The listing builds one solid part. Answer for the finished solid, in the listing's coordinates (mm). A direction names the side the tool comes from. Coordinates: 2 decimals unless noted, no trailing zeros. Order: outer loops, then holes, each group sorted by start corner. A loop starts at its lowest first (then second) coordinate and runs counter-clockwise, first axis right, second up. Notation, with made-up numbers: (-23, -25) -> (18, -25) arc R6 ccw to (18, -19) -> close; hole circle Ø3 at (82.5, 51). An arc over 180 degrees is marked (long way). One line per question, with ' | ' between items.
from build123d import *

# Parameters (mm, degrees)
SKICA1_W                      = 160
SKICA1_H                      = 46
P_IDAT_VYSUNUT_M1_DEPTH       = 1.5
ODEBRAT_VYSUNUT_M1_DEPTH      = 84.254129027
ODEBRAT_VYSUNUT_M1_DEPTH_BACK = 84.254129027
SKICA2_R                      = 1.75
SKICA3_W                      = 10
SKICA3_H                      = 7.5
SKICA3_W_2                    = 7.5
SKICA3_H_2                    = 10
SKICA3_H_3                    = 15
P_IDAT_VYSUNUT_M2_DEPTH       = 10.5
SKICA5_W                      = 6
SKICA5_H                      = 6
P_IDAT_VYSUNUT_M3_DEPTH       = 3.5
SKICA6_R                      = 1.620409531
SKICA6_R_2                    = 1.790047617
SKICA6_R_3                    = 1.76567532
P_IDAT_VYSUNUT_M4_DEPTH       = 8
SKICA7_W                      = 17.5
SKICA7_H                      = 43
SKICA7_W_2                    = 70.5
SKICA7_H_2                    = 30
SKICA7_W_3                    = 40.7
SKICA7_H_3                    = 14
P_IDAT_VYSUNUT_M5_DEPTH       = 15
SKICA8_W                      = 9
SKICA8_H                      = 7.5
P_IDAT_VYSUNUT_M6_DEPTH       = 3.3
SKICA13_W                     = 23.838883278
SKICA13_H                     = 6
SKICA13_W_2                   = 9
SKICA13_H_2                   = 81.2
SKICA13_W_3                   = 7.761116722
P_IDAT_VYSUNUT_M7_DEPTH       = 9.5
SKICA14_W                     = 61
SKICA14_H                     = 30
P_IDAT_VYSUNUT_M8_DEPTH       = 7
SKICA15_W                     = 6
SKICA15_H                     = 30
SKICA15_R                     = 1.75
P_IDAT_VYSUNUT_M9_DEPTH       = 1.7


with BuildPart() as part:
    # Skica1 → Přidat vysunutím1 (new body)
    with BuildSketch(Plane.XY):
        Rectangle(SKICA1_W, SKICA1_H)
    extrude(amount=P_IDAT_VYSUNUT_M1_DEPTH)

    # Skica2 → Odebrat vysunutím1 (cut, two sides: drawn at the far end of the back side and taken through both)
    with BuildSketch(Plane.XY.offset(1.5).offset(-ODEBRAT_VYSUNUT_M1_DEPTH_BACK)):
        with Locations((-71.7, -13.3)):
            Circle(SKICA2_R)
        with Locations((-72.4, 2)):
            Circle(SKICA2_R)
        with Locations((62.7, 3.2)):
            Circle(SKICA2_R)
        with Locations((62.7, -14.6)):
            Circle(SKICA2_R)
    extrude(amount=ODEBRAT_VYSUNUT_M1_DEPTH + ODEBRAT_VYSUNUT_M1_DEPTH_BACK, mode=Mode.SUBTRACT)

    # Skica3 → Přidat vysunutím2 (add)
    with BuildSketch(Plane.XY.offset(1.5)):
        with Locations((-62, -19.25)):
            Rectangle(SKICA3_W, SKICA3_H)
        with Locations((74.25, -8.5)):
            Rectangle(SKICA3_W_2, SKICA3_H_2)
        with Locations((74.25, 9)):
            Rectangle(SKICA3_W_2, SKICA3_H_3)
    extrude(amount=P_IDAT_VYSUNUT_M2_DEPTH)

    # Skica5 → Přidat vysunutím3 (add)
    with BuildSketch(Plane.XY.offset(1.5)):
        with Locations((-62, -8)):
            Rectangle(SKICA5_W, SKICA5_H)
        with Locations((-62, 3)):
            Rectangle(SKICA5_W, SKICA5_H)
        with Locations((-62, 13)):
            Rectangle(SKICA5_W, SKICA5_H)
    extrude(amount=P_IDAT_VYSUNUT_M3_DEPTH)

    # Skica6 → Přidat vysunutím4 (add)
    with BuildSketch(Plane.XY.offset(5)):
        with Locations((-62, 13)):
            Circle(SKICA6_R)
        with Locations((-62, 3)):
            Circle(SKICA6_R_2)
        with Locations((-62, -8)):
            Circle(SKICA6_R_3)
    extrude(amount=P_IDAT_VYSUNUT_M4_DEPTH)

    # Skica7 → Přidat vysunutím5 (add)
    with BuildSketch(Plane.XY.offset(1.5)):
        with Locations((-41.25, 0.5)):
            Rectangle(SKICA7_W, SKICA7_H)
        with Locations((11.75, -6)):
            Rectangle(SKICA7_W_2, SKICA7_H_2)
        with Locations((-3.15, 16)):
            Rectangle(SKICA7_W_3, SKICA7_H_3)
    extrude(amount=P_IDAT_VYSUNUT_M5_DEPTH)

    # Skica8 → Přidat vysunutím6 (add)
    with BuildSketch(Plane.XY.offset(16.5)):
        with Locations((-41.25, 18.25)):
            Rectangle(SKICA8_W, SKICA8_H)
    extrude(amount=P_IDAT_VYSUNUT_M6_DEPTH)

    # Skica13 → Přidat vysunutím7 (add)
    with BuildSketch(Plane.XY.offset(16.5)):
        with Locations((29.119441639, 16.761519328)):
            Rectangle(SKICA13_W, SKICA13_H)
        with Locations((45.538883278, 16.761519328)):
            Rectangle(SKICA13_W_2, SKICA13_H)
        with Locations((45.538883278, 60.361519328)):
            Rectangle(SKICA13_W_2, SKICA13_H_2)
        with Locations((13.319441639, 16.761519328)):
            Rectangle(SKICA13_W_3, SKICA13_H)
    extrude(amount=P_IDAT_VYSUNUT_M7_DEPTH)

    # Skica14 → Přidat vysunutím8 (add)
    with BuildSketch(Plane.XY.offset(16.5)):
        with Locations((14.5, -6)):
            Rectangle(SKICA14_W, SKICA14_H)
    extrude(amount=P_IDAT_VYSUNUT_M8_DEPTH)

    # Skica15 → Přidat vysunutím9 (add)
    # profile 1 of 2: a face of its own
    with BuildSketch(Plane.XY.offset(16.5)):
        with Locations((-26.5, -6)):
            Rectangle(SKICA15_W, SKICA15_H)
        with Locations((-26.5, -18)):
            Circle(SKICA15_R, mode=Mode.SUBTRACT)
        with Locations((-26.5, 6.2)):
            Circle(SKICA15_R, mode=Mode.SUBTRACT)
        with Locations((-26.5, -9)):
            Circle(SKICA15_R, mode=Mode.SUBTRACT)
        with Locations((-26.5, -2.8)):
            Circle(SKICA15_R, mode=Mode.SUBTRACT)
    # profile 2 of 2: a face of its own
    with BuildSketch(Plane.XY.offset(16.5)):
        with Locations((50, -6)):
            Rectangle(SKICA15_W, SKICA15_H)
        with Locations((50, -18)):
            Circle(SKICA15_R, mode=Mode.SUBTRACT)
        with Locations((50, -9)):
            Circle(SKICA15_R, mode=Mode.SUBTRACT)
        with Locations((50, -2.8)):
            Circle(SKICA15_R, mode=Mode.SUBTRACT)
        with Locations((50, 6.2)):
            Circle(SKICA15_R, mode=Mode.SUBTRACT)
    extrude(amount=-P_IDAT_VYSUNUT_M9_DEPTH)


solid = part.part
Item 1: Find the intervals of material crossed by L1, parallel to Y at x = -26.5, z = 15.8; L2, parallel to Y at x = -71.7, z = 0.6; L3, parallel to Z at x = -12, y = 2.5, in increasing order.
Computed values:
L1: y = -21 to -19.75, -16.25 to -10.75, -7.25 to -4.55, -1.05 to 4.45, 7.95 to 9 | L2: y = -23 to -15.05, -11.55 to 0.4, 3.6 to 23 | L3: z = 0 to 23.5
Item 2: Each of these flat-tipped pins is pushed along its axis until it touches: pin 1 Ø3 at (x, z) = (-47, 22) entering from +Y; pin 2 Ø10 at (y, z) = (0, 15) entering from -X; pin 3 Ø5 at (x, y) = (-38, -1.5) entering from +Z; pin 4 Ø5 at (x, y) = (49, 57.5) entering from -Z. Where does it stop, or does it pass through?
Computed values:
pin 1: passes through | pin 2: stops at x = -63.79 | pin 3: stops at z = 16.5 | pin 4: stops at z = 16.5
Item 3: Section A-A, the plane z = 9 is taken. Give the vertices of the cut face in (x, y), plus the area to 3 significant figures.
Computed values:
outline: (-67, -23) -> (-57, -23) -> (-57, -15.5) -> (-67, -15.5) -> close; circle Ø3.58 at (-62, 3); circle Ø3.53 at (-62, -8); circle Ø3.24 at (-62, 13); (-50, -21) -> (-32.5, -21) -> (-32.5, 22) -> (-50, 22) -> close; (-23.5, -21) -> (47, -21) -> (47, 9) -> (17.2, 9) -> (17.2, 23) -> (-23.5, 23) -> close; (70.5, -13.5) -> (78, -13.5) -> (78, -3.5) -> (70.5, -3.5) -> close; (70.5, 1.5) -> (78, 1.5) -> (78, 16.5) -> (70.5, 16.5) -> close | area: 3,730 mm^2
Item 4: Section B-B, the plane y = 65 is taken. Give the vertices of the cut face in (x, z), plus the area to 3 significant figures.
Computed values:
outline: (41.04, 16.5) -> (50.04, 16.5) -> (50.04, 26) -> (41.04, 26) -> close | area: 85.5 mm^2
Item 5: Determine the mould class of faces 6 (the face through (-60.503, 12.379, 8.944)), 7 (the face through (74, 1.5, 7)) for opening direction X: pulls with the +X half, pulls with the -X half, needs draft (parallel to the pull), parting line crosses it, or undercut.
Computed values:
face 6: undercut | face 7: needs draft
Item 6: For faces 1 (the face through (74, -3.5, 7)), 2 (the face through (74, -13.5, 7)), 3 (the face through (-60.293, 3.538, 8.944)), 4 (the face through (70.5, -9, 7)), 5 (the face through (-62, -5, 3)), determine the directions among +Z, -Z, +X, -X, +Y, -Y from which every point of the face is accessible in a straight line to the end or side of a thin tool.
Computed values:
face 1: +Z, +X | face 2: +Z, +X, -Y | face 3: +Z | face 4: +Z, +Y, -Y | face 5: +Z, -X
